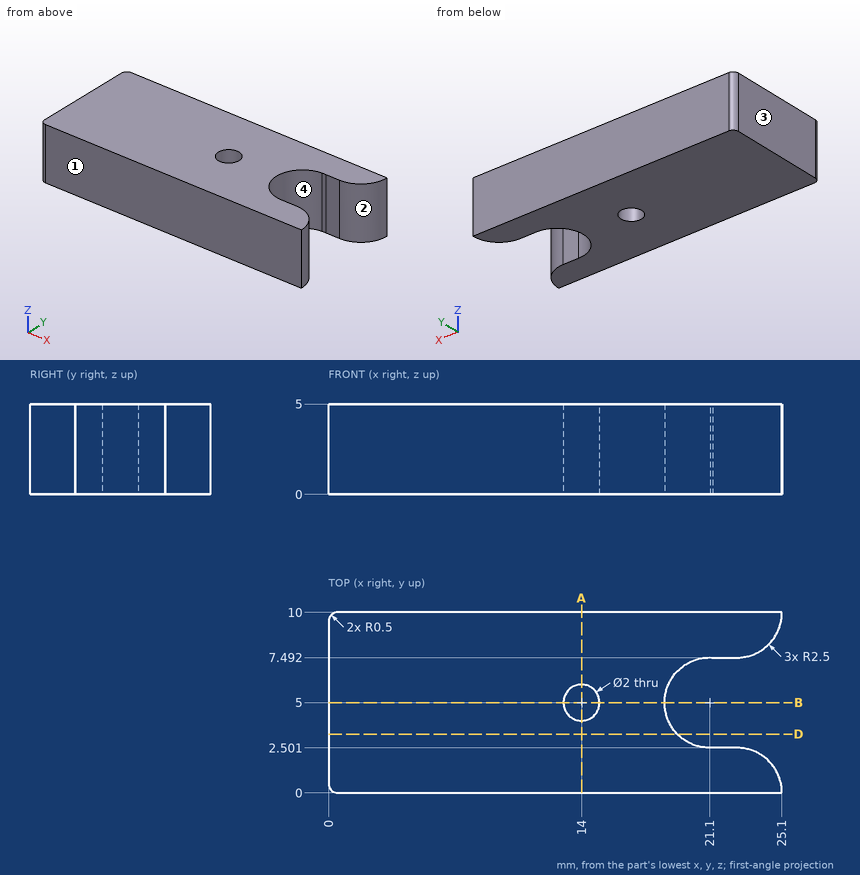
Study the drawing (mm; zero at the part's minimum x, y, z) and answer. Round coordinates to 2 decimals unless told otherwise and drop trailing zeros. Loops run counter-clockwise (first coordinate to the right, second up) from the corner with the lowest first, then second, coordinate; pieces in that order, holes last.
Q1. For a pull along Y with two mould halves and no side action, classify the marked faces 1, 2, 3 and 4 as released by +Y, released by -Y, zero draft, split by the parting line, or undercut.
Q2. Section A-A, the plane x = 14 is taken. Determine the outline of the cut face in (y, z), then the cut area to 3 significant figures.
Q3. Section B-B, the plane y = 5 is taken. Determine the outline of the cut face in (x, z), then the cut area to 3 significant figures.
Q4. Section D-D, the plane y = 3.25 is taken. Determine the outline of the cut face in (x, z) (1 decimal).
Q5. Find the intervals of material crossed by line 1 (Y direction, x = 14, z = 3.5); line 2 (Y direction, x = 19.25, z = 2.5); line 3 (X direction, y = 9.5, z = 0.9), in increasing order.
Q6. Given pin 1 Ø2 at (y, z) = (4, 2) entering from +X; pin 2 Ø1.6 at (x, y) = (14, 5) entering from -Z, each flat-ended and moving along its own axis, determine where each tip first touches the part or whether it passes through.
Completed:
1. face 1: released by -Y
1. face 2: undercut
1. face 3: zero draft
1. face 4: undercut
2. outline: (0, 0) - (4, 0) - (4, 5) - (0, 5) - close; (6, 0) - (10, 0) - (10, 5) - (6, 5) - close
2. area: 40.0 mm2
3. outline: (0, 0) - (13, 0) - (13, 5) - (0, 5) - close; (15, 0) - (18.6, 0) - (18.6, 5) - (15, 5) - close
3. area: 83.0 mm2
4. outline: (0, 0) - (19.3, 0) - (19.3, 5) - (0, 5) - close
5. line 1: y = 0 to 4, 6 to 10
5. line 2: y = 0 to 3.32, 6.68 to 10
5. line 3: x = 0 to 25.05
6. pin 1: stops at x = 19.6
6. pin 2: passes through
